Verification items for the finished model (mm, model axes). A direction names the side the tool comes from. Coordinates: 2 decimals unless noted, no trailing zeros. Order: outer loops, then holes, each group sorted by start corner. A loop starts at its lowest first (then second) coordinate and runs counter-clockwise, first axis right, second up. Notation, with made-up numbers: M 50.5,59 L 89.5,59 A29 ccw 89.5,98 Z; hole C 53,88.25 d4. An arc over 180 degrees is marked long. Answer as a JSON object with one key per item and string values. Group by question number.
(1) Mould release check, pull along Y, two halves, no side actions. Record for faces 1 (the face through (96.459, -26.878, -83.816)), 2 (the face through (77, -42.164, -111)), 3 (the face through (89, -11, -80.2)): released by +Y, released by -Y, zero draft, split by the parting line, or undercut.
(2) Gauge pin test, flat ends, axial feed: pin 1 Ø25 at (y, z) = (-21.08, -92.9) entering from -X; pin 2 Ø6 at (x, y) = (37, -16.5) entering from +Z. Record the tip position at first contact, or that the pin passes through.
(3) Material ranges on line 1 (Y direction, x = 88.9, z = -88.25); line 2 (X direction, y = -3, z = -97.5); line 3 (Z direction, x = 13, y = -17.5), recorded low to high.
(4) Cross-section at C-C (y = -26). Enter the section's corners in (x, z).
(5) Access from +Z, -Z, +X, -X, +Y, -Y to the whole of each face (thin tool, end or side, straight path). Record for faces 4 (the face through (50.8, -11, -93)), 5 (the face through (63, -21, -131)).
(6) Cross-section at A-A (z = -88). Enter the section's corners in (x, y) (3 decimals).
(7) Cross-section at D-D (x = 85). Enter the section's corners in (y, z) (3 decimals).
(8) Cross-section at B-B (x = 108). Enter the section's corners in (y, z) (3 decimals).
from build123d import *

# Parameters (mm, degrees)
F1_DEPTH = 42.164
F3_D     = 19.05
F5_D     = 19.05


with BuildPart() as f1:
    # F0 (on Front) → F1 (new body)
    with BuildSketch(Plane.XZ):
        Polygon((127, -80.199791), (50.8, -80.199791), (50.8, -105.599791), (0, -105.599791), (0, -130.999791), (127, -130.999791), align=None)
    extrude(amount=F1_DEPTH)

    # F3 (through all)
    with Locations(Plane(origin=(50.8, 0, 0), x_dir=(0, -1, 0), z_dir=(-1, 0, 0))):
        with Locations((21.082, -92.899791)):
            Hole(F3_D / 2)

    # F5 (through all)
    with Locations(Plane.XY.offset(-80.199791)):
        with Locations((88.9, -21.082)):
            Hole(F5_D / 2)


solid = f1.part
Taken from the geometry:
{
 "1": {"face 1": "undercut", "face 2": "released by -Y", "face 3": "zero draft"},
 "2": {"pin 1": "stops at x = 50.8", "pin 2": "stops at z = -105.6"},
 "3": {"line 1": "y = -42.16 to -30.61, -11.56 to 0", "line 2": "x = 50.8 to 127", "line 3": "z = -131 to -105.6"},
 "4": {"outline": "M 0,-131 L 80.74,-131 L 80.74,-101.06 L 50.8,-101.06 L 50.8,-105.6 L 0,-105.6 Z; M 50.8,-84.74 L 80.74,-84.74 L 80.74,-80.2 L 50.8,-80.2 Z; M 97.06,-131 L 127,-131 L 127,-101.06 L 97.06,-101.06 Z; M 97.06,-84.74 L 127,-84.74 L 127,-80.2 L 97.06,-80.2 Z"},
 "5": {"face 4": "+Z, -X, +Y, -Y", "face 5": "-Z, +X, -X, +Y, -Y"},
 "6": {"outline": "M 50.8,-42.164 L 127,-42.164 L 127,-29.25 L 93.8,-29.25 A9.525 cw 84,-29.25 L 50.8,-29.25 Z; M 50.8,-12.914 L 84,-12.914 A9.525 cw 93.8,-12.914 L 127,-12.914 L 127,0 L 50.8,0 Z"},
 "7": {"outline": "M -42.164,-131 L -29.772,-131 L -29.772,-96.8 A9.525 cw -29.772,-89 L -29.772,-80.2 L -42.164,-80.2 Z; M -12.392,-131 L 0,-131 L 0,-80.2 L -12.392,-80.2 L -12.392,-89 A9.525 cw -12.392,-96.8 Z"},
 "8": {"outline": "M -42.164,-131 L 0,-131 L 0,-80.2 L -42.164,-80.2 Z; hole C -21.082,-92.9 d19.05"}
}
